Autodesk Inventor part; units mm, degrees
ref_plane "YZ Plane" through (0, 0, 0) normal (1, 0, 0) x (0, 1, 0)
ref_plane "XZ Plane" through (0, 0, 0) normal (0, 1, 0) x (-1, 0, 0)
ref_plane "XY Plane" through (0, 0, 0) normal (0, 0, 1) x (1, 0, 0)
sketch "スケッチ1" plane through (0, 0, 0) normal (0, 0, 1) x (1, 0, 0)
  circle A0 centre (0, 0) radius 10.5
  circle A1 centre (0, 0) radius 4
  dimension "d0" = 21
  dimension "d1" = 8
extrude "押し出し1" add sketch "スケッチ1" along normal blind 3.5
sketch "スケッチ2" plane through (0, 0, 3.5) normal (0, 0, 1) x (1, 0, 0)
  line L0 (0, 0) -> (0, 10.5) construction
  circle A0 centre (0, 0) radius 10.5
  point P0 (0, 8.5)
  point P1 (-6.0104, 6.0104)
  point P2 (-8.5, 0)
  point P3 (-6.0104, -6.0104)
  point P4 (0, -8.5)
  point P5 (6.0104, -6.0104)
  point P6 (8.5, 0)
  point P7 (6.0104, 6.0104)
  dimension "d4" = 8.5
  dimension "d7" = 360
hole "穴1" at (0, 8.5, 3.5) at (-6.0104, 6.0104, 3.5) at (-8.5, 0, 3.5) at (-6.0104, -6.0104, 3.5) at (0, -8.5, 3.5) at (6.0104, -6.0104, 3.5) at (8.5, 0, 3.5) at (6.0104, 6.0104, 3.5) direction (0, 0, -1) diameter 2.113 end through all
properties part number "free_horn" material "アルミニウム 6061"
CAD build for the part. Positions are in the model's coordinates, mm. Round coordinates to 2 decimals unless told otherwise and drop trailing zeros. Order: outer loops, then holes, each group sorted by start corner. A loop starts at its lowest first (then second) coordinate and runs counter-clockwise, first axis right, second up. Notation, with made-up numbers: M -20,35.5 L -5,35.5 A17 ccw -5,53.5 Z; hole C 11.25,46.5 d9. An arc over 180 degrees is marked long. Use one line per item in the form item = value.
Q1. Probe L1, parallel to Y at x = 0, z = 2; L2, parallel to Y at x = 0.25, z = 2; L3, parallel to X at y = 0.75, z = 0.9. List the from-to ranges inside material, lowest first.
Recorded:
L1 = -10.5 to -9.56, -7.44 to -4, 4 to 7.44, 9.56 to 10.5
L2 = -10.5 to -9.53, -7.47 to -3.99, 3.99 to 7.47, 9.53 to 10.5
L3 = -10.47 to -9.24, -7.76 to -3.93, 3.93 to 7.76, 9.24 to 10.47
Q2. Flat gauge pins, fed straight in: P1, Ø3.5, axis at x = 8.5, y = 0, coming from the +Z side; P2, Ø2, axis at y = 5, z = 2.5, coming from the +X side. Where does each tip first touch, or does it go through?
Recorded:
P1 = 3.5
P2 = 9.71
Q3. Two-plate mould, pull along Y, no slides. Class faces 1 (the cylindrical face through (-0.046, -7.445, 1.726)), 2 (the flat face through (5, 0, 0)), 3 (the cylindrical face through (10, -3.2, 1.7)), 4 (the cylindrical face through (-6.328, -7.018, 1.726)): +Y half, -Y half, draft (parallel to the pull), parting line (faces both ways), or undercut.
Recorded:
face_1 = undercut
face_2 = draft
face_3 = parting line
face_4 = undercut
Q4. Saw through at D-D on z = 2.2. State how many separate pieces and enclosed holes the cut face has, then the cut area to 3 significant figures.
Recorded:
separate_pieces = 1
enclosed_holes = 9
area = 268 mm^2
Q5. Saw through at B-B on y = 1.5. Give the cut face in (x, z), then the cut area to 3 significant figures.
Recorded:
outline = M -10.39,0 L -3.71,0 L -3.71,3.5 L -10.39,3.5 Z; M 3.71,0 L 10.39,0 L 10.39,3.5 L 3.71,3.5 Z
area = 46.8 mm^2
Q6. Saw through at A-A on x = 0. Give the cut face in (y, z), then the cut area to 3 significant figures.
Recorded:
outline = M -10.5,0 L -9.56,0 L -9.56,3.5 L -10.5,3.5 Z; M -7.44,0 L -4,0 L -4,3.5 L -7.44,3.5 Z; M 4,0 L 7.44,0 L 7.44,3.5 L 4,3.5 Z; M 9.56,0 L 10.5,0 L 10.5,3.5 L 9.56,3.5 Z
area = 30.7 mm^2
Q7. Saw through at C-C on x = -2.5. Give the cut face in (y, z).
Recorded:
outline = M -10.2,0 L -3.12,0 L -3.12,3.5 L -10.2,3.5 Z; M 3.12,0 L 10.2,0 L 10.2,3.5 L 3.12,3.5 Z
